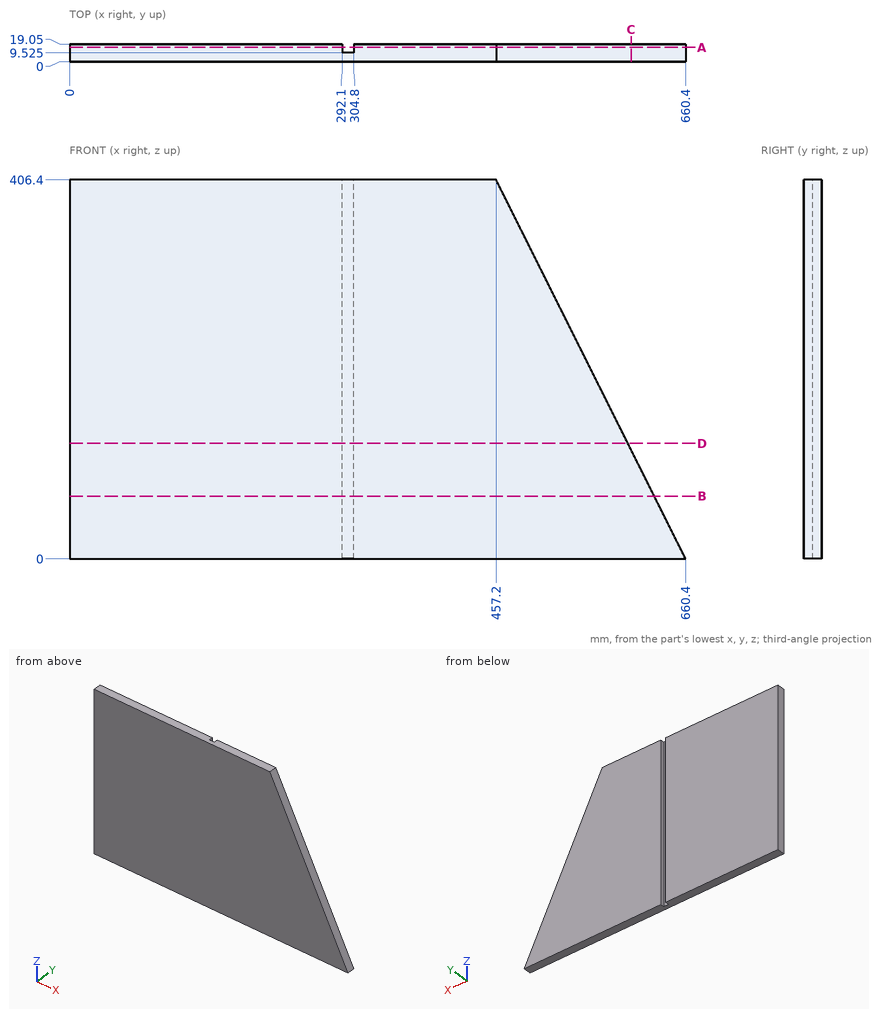
Verification items for this drawing (mm, ordinates from the low corner). Give positions to 0.01 mm unless a question says otherwise; leave off trailing zeros. Loops run counter-clockwise (first coordinate to the right, second up) from the corner with the lowest first, then second, coordinate; pieces in that order, holes last. Notation, with made-up numbers: M 76.25,-6.5 L 102.25,-6.5 A21 cw 102.25,25.5 Z; hole C -25,53 d8. An arc over 180 degrees is marked long. Answer as a JSON object with one key per item and string values. Group by question number.
Q1. Cross-section at B-B on z = 67.5. Record the cut outline in (x, y) (3 decimals).
Q2. Cross-section at A-A on y = 15.5. Record the cut outline in (x, z), then the cut area to 3 significant figures.
Q3. Cross-section at C-C on x = 602. Record the cut outline in (y, z).
Q4. Cross-section at D-D on z = 124. Record the cut outline in (x, y) (3 decimals), then the cut area to 3 significant figures.
Q5. Material ranges on line 1 along X through (y, z) = (14.5, 257); line 2 along X through (y, z) = (15.5, 122); line 3 along Z through (x, y) = (632, 2), recorded low to high. Write a range as [from, to].
Q6. Go/stop test with flat-tipped pins: P1, Ø6, axis at y = 16.5, z = 160, coming from the +X side; P2, Ø4, axis at x = 298, z = 157.5, coming from the +Y side (3 decimals); P3, Ø3, axis at x = 542, y = 14, coming from the +Z side. Record where each tip stops, or that it passes through.
Evaluation:
{
 "1": {"outline": "M 0,0 L 626.65,0 L 626.65,19.05 L 304.8,19.05 L 304.8,9.525 L 292.1,9.525 L 292.1,19.05 L 0,19.05 Z"},
 "2": {"outline": "M 0,0 L 292.1,0 L 292.1,406.4 L 0,406.4 Z; M 304.8,0 L 660.4,0 L 457.2,406.4 L 304.8,406.4 Z", "area": "222,000 mm2"},
 "3": {"outline": "M 0,0 L 19.05,0 L 19.05,116.8 L 0,116.8 Z"},
 "4": {"outline": "M 0,0 L 598.4,0 L 598.4,19.05 L 304.8,19.05 L 304.8,9.525 L 292.1,9.525 L 292.1,19.05 L 0,19.05 Z", "area": "11,300 mm2"},
 "5": {"line 1": "x = [0, 292.1], [304.8, 531.9]", "line 2": "x = [0, 292.1], [304.8, 599.4]", "line 3": "z = [0, 56.8]"},
 "6": {"P1": "stops at x = 581.9", "P2": "stops at y = 9.525", "P3": "stops at z = 239.8"}
}
